Model file for the job. Use its own axes, mm. Face numbers are marked on the shaded views. A direction names the side the tool comes from. Coordinates: 2 decimals unless noted, no trailing zeros. Write each loop counter-clockwise with the first axis right and the second up, starting at its lowest first coordinate (ties: lowest second). Pieces come first, ordered by that corner, then holes. Notation, with made-up numbers: (69.5, -13.75) -> (128.5, -13.75) arc R13 ccw to (128.5, -1.75) -> close; hole circle Ø6 at (-25, -13.75). An arc over 180 degrees is marked (long way). Answer as a JSON object with one key per item and string values. Group by question number.
from build123d import *

# Parameters (mm, degrees)
F0_W         = 1500
F0_H         = 150
F1_DEPTH     = 56.30659
F2_W         = 1500
F2_H         = 150
F2_W_2       = 300.6279
F2_H_2       = 120
F3_DEPTH     = 130
F6_D         = 20
F6_DEPTH     = 16.486247664
F7_D         = 20
F8_T1_DEPTH  = 887.8761290407
F9_W         = 186.30659
F9_H         = 25
F10_DEPTH    = 80
F11_T1_DEPTH = 543.3223571193
F11_T3_DEPTH = 543.3223571193
F13_D        = 20


# Not quite as in the source:
# - a fillet or chamfer that OpenCascade refuses, or shapes differently, is made with other operations: its cross-section is extruded or revolved along the edge and cut away or added
# - a feature names something its author has since deleted; it is built from what else it names


with BuildPart() as f1:
    # F0 (on Front) → F1 (new body)
    with BuildSketch(Plane.XZ):
        with Locations((295.444762387, 72.4433880299)):
            Rectangle(F0_W, F0_H)
    extrude(amount=F1_DEPTH)

    # F2 (on face) → F3 (join)
    with BuildSketch(Plane.XZ.offset(56.30659)):
        with Locations((295.444762387, 72.4433880299)):
            Rectangle(F2_W, F2_H)
        with Locations((-104.6067848625, 70.9581403659)):
            Rectangle(F2_W_2, F2_H_2, mode=Mode.SUBTRACT)
    extrude(amount=F3_DEPTH)

    # F6 (through all, one way)
    with BuildSketch(Plane(origin=(0, 0, 130.9581403659), x_dir=(1, 0, 0), z_dir=(0, 0, -1))):
        with Locations((-96.1152985692, 143.3657854795)):
            Circle(F6_D / 2)
    extrude(amount=-F6_DEPTH, mode=Mode.SUBTRACT)

    # F7 (through all)
    with Locations(Plane(origin=(0, 0, -2.5566119701), x_dir=(1, 0, 0), z_dir=(0, 0, -1))):
        with Locations((-96.1604490876, 143.5462683439)):
            Hole(F7_D / 2)

    # F8: fillet of radius 147.5752258081 on 2 edges, made by hand

    # F8_s2 → F8_t1 (cut)
    with BuildSketch(Plane.XY.offset(-371.4946764904)):
        with BuildLine():
            ThreePointArc((-454.555237613, -38.7313641919), (-411.331454709, -143.0828070959), (-306.9800118049, -186.30659))
            Line((-306.9800118049, -186.30659), (-454.555237613, -186.30659))
            Line((-454.555237613, -186.30659), (-454.555237613, -38.7313641919))
        make_face()
        with BuildLine():
            ThreePointArc((-306.9800118049, 0), (-411.331454709, -43.2237829041), (-454.555237613, -147.5752258081))
            Line((-454.555237613, -147.5752258081), (-454.555237613, 0))
            Line((-454.555237613, 0), (-306.9800118049, 0))
        make_face()
    extrude(amount=F8_T1_DEPTH, mode=Mode.SUBTRACT)

    # F9 (on face) → F10 (join)
    with BuildSketch(Plane.YZ.offset(1045.444762387)):
        with Locations((-93.153295, 134.9433880299)):
            Rectangle(F9_W, F9_H)
        with Locations((-93.153295, 9.9433880299)):
            Rectangle(F9_W, F9_H)
    extrude(amount=F10_DEPTH)

    # F11: fillet of radius 103.6644714239 on 4 edges, made by hand

    # F11_s2 → F11_t1 (cut)
    with BuildSketch(Plane.XY.offset(-136.7177905297)):
        with BuildLine():
            ThreePointArc((1125.444762387, -103.6644714239), (1095.082141675, -30.3626207119), (1021.7802909631, 0))
            Line((1021.7802909631, 0), (1125.444762387, 0))
            Line((1125.444762387, 0), (1125.444762387, -103.6644714239))
        make_face()
        with BuildLine():
            ThreePointArc((1021.7802909631, -186.30659), (1095.082141675, -155.9439692881), (1125.444762387, -82.6421185761))
            Line((1125.444762387, -82.6421185761), (1125.444762387, -186.30659))
            Line((1125.444762387, -186.30659), (1021.7802909631, -186.30659))
        make_face()
    extrude(amount=F11_T1_DEPTH, mode=Mode.SUBTRACT)

    # F11_s4 → F11_t3 (cut)
    with BuildSketch(Plane.XY.offset(-261.7177905297)):
        with BuildLine():
            ThreePointArc((1125.444762387, -103.6644714239), (1095.082141675, -30.3626207119), (1021.7802909631, 0))
            Line((1021.7802909631, 0), (1125.444762387, 0))
            Line((1125.444762387, 0), (1125.444762387, -103.6644714239))
        make_face()
        with BuildLine():
            ThreePointArc((1021.7802909631, -186.30659), (1095.082141675, -155.9439692881), (1125.444762387, -82.6421185761))
            Line((1125.444762387, -82.6421185761), (1125.444762387, -186.30659))
            Line((1125.444762387, -186.30659), (1021.7802909631, -186.30659))
        make_face()
    extrude(amount=F11_T3_DEPTH, mode=Mode.SUBTRACT)

    # F13 (through all)
    with Locations(Plane(origin=(0, 0, -2.5566119701), x_dir=(1, 0, 0), z_dir=(0, 0, -1))):
        with Locations((1096.6192483902, 92.0223891735)):
            Hole(F13_D / 2)


solid = f1.part
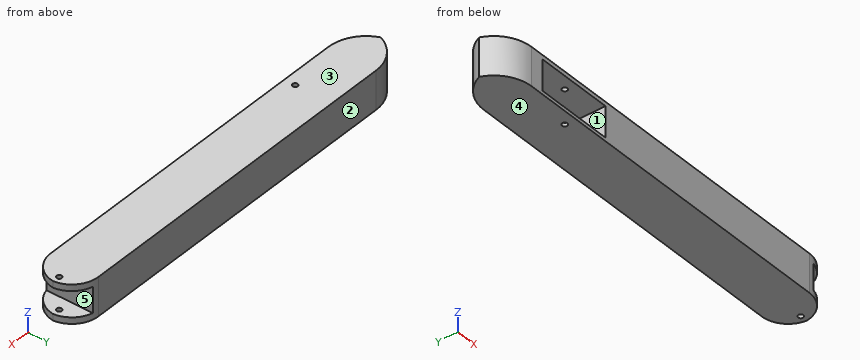
(1) Pull direction Z, two halves, no side cores. Call the marked faces 3, 4 and 5: released by +Z, released by -Z, zero draft, split by the parting line, or undercut.
(2) Cut at A-A on z = 52. List the corners of the cut face in (x, y), plus the area to 3 significant figures.
(3) Wall check: probe 1 along Z at (x, y) = (-185.5, -117); probe 2 along X at (y, z) = (-70, 51); probe 3 along X at (y, z) = (-60, 112.5). Give the ranges that are in metal, low to high.
(4) 3-axis set-ups, long thin cutter, end or side, ignore diameter. For the marked faces 1 and 2: which of +Z, -Z, +X, -X, +Y, -Y reach the whole face in a straight line?
(5) Cut at B-B on y = -120. List the corners of the cut face in (x, z).
(6) Cut at C-C on y = -41. List the corners of the cut face in (x, z).
(7) Pin check, flat tips, straight feed: pin 1 (3 mm diameter, centred on y = -139.5, z = 13.5, fed in from +X); pin 2 (4 mm diameter, centred on y = -68, z = 36.5, fed in from -X); pin 3 (5 mm diameter, centred on y = -75.5, z = 92.5, fed in from -X); pin 4 (16 mm diameter, centred on x = -96.16, y = -143.55, fed in from -Z). Stop position of each tip, or through.
Results found:
{
 "1": {"face 3": "released by +Z", "face 4": "released by -Z", "face 5": "undercut"},
 "2": {"outline": "(-444.15, -93.15) arc R147.58 ccw to (-306.98, -186.31) -> (-254.92, -186.31) -> (-254.92, -56.31) -> (45.71, -56.31) -> (45.71, -186.31) -> (1021.78, -186.31) arc R103.66 ccw to (1045.44, -183.57) -> (1045.44, -2.74) arc R103.66 ccw to (1021.78, 0) -> (-306.98, 0) arc R147.58 ccw to start", "area": "231,000 mm²"},
 "3": {"probe 1": "z = -2.56 to 10.96, 130.96 to 147.44", "probe 2": "x = -432.52 to -254.92, 45.71 to 1045.44", "probe 3": "x = -425.76 to -254.92, 45.71 to 1045.44"},
 "4": {"face 1": "-Y", "face 2": "+Z, -Z, +X, -X, +Y"},
 "5": {"outline": "(-430.16, -2.56) -> (1118.48, -2.56) -> (1118.48, 22.44) -> (1045.44, 22.44) -> (1045.44, 122.44) -> (1118.48, 122.44) -> (1118.48, 147.44) -> (-430.16, 147.44) -> close; hole (-254.92, 10.96) -> (45.71, 10.96) -> (45.71, 130.96) -> (-254.92, 130.96) -> close"},
 "6": {"outline": "(-409.06, -2.56) -> (1104.36, -2.56) -> (1104.36, 22.44) -> (1045.44, 22.44) -> (1045.44, 122.44) -> (1104.36, 122.44) -> (1104.36, 147.44) -> (-409.06, 147.44) -> close"},
 "7": {"pin 1": "stops at x = 1109.43", "pin 2": "stops at x = -432.52", "pin 3": "stops at x = -437.13", "pin 4": "passes through"}
}
